The model under review builds one solid part; all positions refer to its coordinate system, in mm. Face numbers are marked on the shaded views. Coordinates: 2 decimals unless noted, no trailing zeros. Loops run counter-clockwise (first coordinate to the right, second up) from the corner with the lowest first, then second, coordinate; pieces in that order, holes last. Notation, with made-up numbers: (47, 83) - (65, 83) arc R13 cw to (65, 96) - close; hole circle Ø4 at (89.5, -3). An arc over 180 degrees is marked (long way). Answer in a Markdown table with one row per item. Add a question column.
(1) For P1, Ø5, axis at x = 28, z = 2.5, coming from the +Y side; P2, Ø4, axis at x = 67.5, y = 2.5, coming from the -Z side; P3, Ø2.5, axis at x = 20.5, y = 3, coming from the -Z side, all flat-tipped, find the tip position at first contact; note any pin that passes through.
(2) We need section B-B on x = 18. Write out the cut boundary in (y, z), plus the area to 3 significant figures.
(3) We need section A-A on z = -55. Write out the cut boundary in (x, y), plus the area to 3 significant figures.
(4) For line 1 along X through (y, z) = (0.75, -34); line 2 along X through (y, z) = (7, 6.5); line 3 along Y through (x, z) = (31.5, -3.5), list the stretches that pass through material, from the lowest coordinate up.
(5) Mouldability with a two-part tool opening along X and no side actions: class the marked faces 1 and 2 as +X half, -X half, draft (parallel to the pull), parting line (faces both ways), or undercut.
from build123d import *

# Parameters (mm, degrees)
EXTRUDE_4_DEPTH     = 5.6
EXTRUDE_4_2_DEPTH   = 5.6
SKETCH_9_W          = 2.6
SKETCH_9_H          = 12.4
SKETCH_9_H_2        = 50
EXTRUDE_6_DEPTH     = 2.6
DS18B20_W           = 5
DS18B20_H           = 42.5
DS18B20_H_2         = 10.1
CUT_EXTRUDE_1_DEPTH = 5
SKETCH_7_W          = 1.5
SKETCH_7_H          = 75
EXTRUDE_8_DEPTH     = 2.2
FILLET_1_RADIUS     = 4.7
FILLET_1_LENGTH     = 3
FILLET_2_R          = 7.3
FILLET_3_RADIUS     = 4.7
FILLET_3_LENGTH     = 3
FILLET_4_R          = 7.3
FILLET_5_RADIUS     = 4.7
FILLET_5_LENGTH     = 3
FILLET_6_R          = 7.3
FILLET_7_R          = 7.3
FILLET_8_RADIUS     = 4.7
FILLET_8_LENGTH     = 3
FILLET_9_RADIUS     = 4.7
FILLET_9_LENGTH     = 3
FILLET_10_R         = 7.3


with BuildPart() as part:
    # Sketch 2111 → Extrude 4 (new body)
    with BuildSketch(Plane(origin=(0, 0, 0), x_dir=(1, 0, 0), z_dir=(0, 1, 0))):
        Polygon((14.6, 50), (14.6, 0), (24, 0), (24, 50), (24, 52.6), (38.6, 52.6), (38.6, 50), (38.6, 0), (48, 0), (48, 50), (48, 52.6), (62.6, 52.6), (62.6, 50), (62.6, 0), (62.6, -12.4), (74.6, -12.4), (74.6, 62.6), (-12, 62.6), (-12, -12.4), (0, -12.4), (0, 0), (0, 50), (0, 52.6), (14.6, 52.6), align=None)
    extrude(amount=EXTRUDE_4_DEPTH)



with BuildPart() as body_2:
    # Sketch 2111 → Extrude 4 2 (new body)
    with BuildSketch(Plane(origin=(0, 0, 0), x_dir=(1, 0, 0), z_dir=(0, 1, 0))):
        Polygon((12, -2.6), (12, 0), (12, 50), (2.6, 50), (2.6, 0), (2.6, -12.4), (60, -12.4), (60, 0), (60, 50), (50.6, 50), (50.6, 0), (50.6, -2.6), (36, -2.6), (36, 0), (36, 50), (26.6, 50), (26.6, 0), (26.6, -2.6), align=None)
    extrude(amount=EXTRUDE_4_2_DEPTH)


with BuildPart() as part_1:
    add(part.part)

    add(body_2.part)  # Extrude 6 merges body 2
    # Sketch 9 → Extrude 6 (add)
    with BuildSketch(Plane(origin=(0, 0, 0), x_dir=(1, 0, 0), z_dir=(0, 1, 0))):
        with Locations((1.3, -6.2)):
            Rectangle(SKETCH_9_W, SKETCH_9_H)
        with Locations((1.3, 25)):
            Rectangle(SKETCH_9_W, SKETCH_9_H_2)
        Polygon((14.6, 0), (12, 0), (12, -2.6), (26.6, -2.6), (26.6, 0), (24, 0), align=None)
        with Locations((13.3, 25)):
            Rectangle(SKETCH_9_W, SKETCH_9_H_2)
        with Locations((25.3, 25)):
            Rectangle(SKETCH_9_W, SKETCH_9_H_2)
        Polygon((2.6, 50), (12, 50), (14.6, 50), (14.6, 52.6), (0, 52.6), (0, 50), align=None)
        Polygon((24, 52.6), (24, 50), (26.6, 50), (36, 50), (38.6, 50), (38.6, 52.6), align=None)
        with Locations((37.3, 25)):
            Rectangle(SKETCH_9_W, SKETCH_9_H_2)
        Polygon((38.6, 0), (36, 0), (36, -2.6), (50.6, -2.6), (50.6, 0), (48, 0), align=None)
        with Locations((49.3, 25)):
            Rectangle(SKETCH_9_W, SKETCH_9_H_2)
        Polygon((50.6, 50), (60, 50), (62.6, 50), (62.6, 52.6), (48, 52.6), (48, 50), align=None)
        with Locations((61.3, 25)):
            Rectangle(SKETCH_9_W, SKETCH_9_H_2)
        with Locations((61.3, -6.2)):
            Rectangle(SKETCH_9_W, SKETCH_9_H)
    extrude(amount=EXTRUDE_6_DEPTH)

    # DS18B20 → Cut-Extrude 1 (cut)
    with BuildSketch(Plane(origin=(0, 5.6, 0), x_dir=(1, 0, 0), z_dir=(0, 1, 0))):
        Polygon((-8.5, 62.6), (-8.5, 17.457748372), (-3.5, 19.012014035), (-3.5, 62.6), align=None)
        Polygon((-3.5, 19.012014035), (-8.5, 17.457748372), (-8.5, 10), (-3.5, 10), align=None)
        with Locations((19.3, 41.35)):
            Rectangle(DS18B20_W, DS18B20_H)
        with Locations((19.3, 15.05)):
            Rectangle(DS18B20_W, DS18B20_H_2)
        with Locations((43.3, 41.35)):
            Rectangle(DS18B20_W, DS18B20_H)
        with Locations((43.3, 15.05)):
            Rectangle(DS18B20_W, DS18B20_H_2)
        with Locations((68.6, 41.35)):
            Rectangle(DS18B20_W, DS18B20_H)
        with Locations((68.6, 15.05)):
            Rectangle(DS18B20_W, DS18B20_H_2)
    extrude(amount=-CUT_EXTRUDE_1_DEPTH, mode=Mode.SUBTRACT)

    # Sketch 7 → Extrude 8 (add)
    with BuildSketch(Plane(origin=(0, 5.6, 0), x_dir=(1, 0, 0), z_dir=(0, 1, 0))):
        with Locations((-11.25, 25.1)):
            Rectangle(SKETCH_7_W, SKETCH_7_H)
        with Locations((73.85, 25.1)):
            Rectangle(SKETCH_7_W, SKETCH_7_H)
    extrude(amount=EXTRUDE_8_DEPTH)

    # Fillet 1: full round fillet: the end face becomes a half cylinder, R = half its width
    fillet_1_face = Plane((55.3, 4.1, -50), x_dir=(0, -1, 0), z_dir=(0, 0, -1))  # on the end face: x along it, z out of the body
    fillet_1_slab = fillet_1_face.offset(-FILLET_1_RADIUS / 2) * Box(FILLET_1_LENGTH, 2 * FILLET_1_RADIUS, FILLET_1_RADIUS, mode=Mode.PRIVATE)  # the body's end, R deep
    fillet_1_round = Plane((55.3, 4.1, -45.3), x_dir=(0, 0, -1), z_dir=(0, -1, 0)) * Cylinder(FILLET_1_RADIUS, FILLET_1_LENGTH, mode=Mode.PRIVATE)  # its axis R under the face
    add(fillet_1_slab - fillet_1_round, mode=Mode.SUBTRACT)

    # Fillet 2
    fillet_2_edges = [part_1.edges().sort_by_distance(p)[0] for p in [
        (62.6, 4.1, -52.6),
        (48, 4.1, -52.6),
    ]]
    fillet(fillet_2_edges, radius=FILLET_2_R - 0.0001)  # a hair under: the kernel refuses the full size

    # Fillet 3: full round fillet: the end face becomes a half cylinder, R = half its width
    fillet_3_face = Plane((43.3, 4.1, 0), x_dir=(0, 1, 0), z_dir=(0, 0, 1))  # on the end face: x along it, z out of the body
    fillet_3_slab = fillet_3_face.offset(-FILLET_3_RADIUS / 2) * Box(FILLET_3_LENGTH, 2 * FILLET_3_RADIUS, FILLET_3_RADIUS, mode=Mode.PRIVATE)  # the body's end, R deep
    fillet_3_round = Plane((43.3, 4.1, -4.7), x_dir=(0, 0, 1), z_dir=(0, 1, 0)) * Cylinder(FILLET_3_RADIUS, FILLET_3_LENGTH, mode=Mode.PRIVATE)  # its axis R under the face
    add(fillet_3_slab - fillet_3_round, mode=Mode.SUBTRACT)

    # Fillet 4
    fillet_4_edges = [part_1.edges().sort_by_distance(p)[0] for p in [
        (50.6, 4.1, 2.6),
        (36, 4.1, 2.6),
    ]]
    fillet(fillet_4_edges, radius=FILLET_4_R - 0.0001)  # a hair under: the kernel refuses the full size

    # Fillet 5: full round fillet: the end face becomes a half cylinder, R = half its width
    fillet_5_face = Plane((31.3, 4.1, -50), x_dir=(0, -1, 0), z_dir=(0, 0, -1))  # on the end face: x along it, z out of the body
    fillet_5_slab = fillet_5_face.offset(-FILLET_5_RADIUS / 2) * Box(FILLET_5_LENGTH, 2 * FILLET_5_RADIUS, FILLET_5_RADIUS, mode=Mode.PRIVATE)  # the body's end, R deep
    fillet_5_round = Plane((31.3, 4.1, -45.3), x_dir=(0, 0, -1), z_dir=(0, -1, 0)) * Cylinder(FILLET_5_RADIUS, FILLET_5_LENGTH, mode=Mode.PRIVATE)  # its axis R under the face
    add(fillet_5_slab - fillet_5_round, mode=Mode.SUBTRACT)

    # Fillet 6
    fillet_6_edges = [part_1.edges().sort_by_distance(p)[0] for p in [
        (38.6, 4.1, -52.6),
        (24, 4.1, -52.6),
    ]]
    fillet(fillet_6_edges, radius=FILLET_6_R - 0.0001)  # a hair under: the kernel refuses the full size

    # Fillet 7
    fillet_7_edges = [part_1.edges().sort_by_distance(p)[0] for p in [
        (26.6, 4.1, 2.6),
        (12, 4.1, 2.6),
    ]]
    fillet(fillet_7_edges, radius=FILLET_7_R - 0.0001)  # a hair under: the kernel refuses the full size

    # Fillet 8: full round fillet: the end face becomes a half cylinder, R = half its width
    fillet_8_face = Plane((19.3, 4.1, 0), x_dir=(0, 1, 0), z_dir=(0, 0, 1))  # on the end face: x along it, z out of the body
    fillet_8_slab = fillet_8_face.offset(-FILLET_8_RADIUS / 2) * Box(FILLET_8_LENGTH, 2 * FILLET_8_RADIUS, FILLET_8_RADIUS, mode=Mode.PRIVATE)  # the body's end, R deep
    fillet_8_round = Plane((19.3, 4.1, -4.7), x_dir=(0, 0, 1), z_dir=(0, 1, 0)) * Cylinder(FILLET_8_RADIUS, FILLET_8_LENGTH, mode=Mode.PRIVATE)  # its axis R under the face
    add(fillet_8_slab - fillet_8_round, mode=Mode.SUBTRACT)

    # Fillet 9: full round fillet: the end face becomes a half cylinder, R = half its width
    fillet_9_face = Plane((7.3, 4.1, -50), x_dir=(0, 1, 0), z_dir=(0, 0, -1))  # on the end face: x along it, z out of the body
    fillet_9_slab = fillet_9_face.offset(-FILLET_9_RADIUS / 2) * Box(FILLET_9_LENGTH, 2 * FILLET_9_RADIUS, FILLET_9_RADIUS, mode=Mode.PRIVATE)  # the body's end, R deep
    fillet_9_round = Plane((7.3, 4.1, -45.3), x_dir=(0, 0, -1), z_dir=(0, 1, 0)) * Cylinder(FILLET_9_RADIUS, FILLET_9_LENGTH, mode=Mode.PRIVATE)  # its axis R under the face
    add(fillet_9_slab - fillet_9_round, mode=Mode.SUBTRACT)

    # Fillet 10
    fillet_10_edges = [part_1.edges().sort_by_distance(p)[0] for p in [
        (14.6, 4.1, -52.6),
        (0, 4.1, -52.6),
    ]]
    fillet(fillet_10_edges, radius=FILLET_10_R - 0.0001)  # a hair under: the kernel refuses the full size


solid = part_1.part
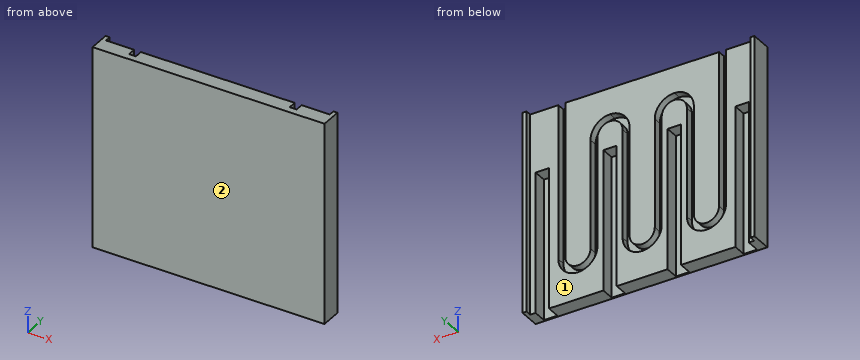
Outcome:
| question | item | result |
|---|---|---|
| 1 | P1 | y = 5.6 |
| 1 | P2 | z = -62.6 |
| 1 | P3 | z = -10 |
| 2 | outline | (0, -62.6) - (0.6, -62.6) - (0.6, -10) - (5.6, -10) - (5.6, -0.18) - (2.6, -0.18) - (2.6, 2.48) - (5.6, 2.48) - (5.6, 12.4) - (0, 12.4) - close |
| 2 | area | 149 mm² |
| 3 | outline | (-12, 0) - (74.6, 0) - (74.6, 7.8) - (73.1, 7.8) - (73.1, 5.6) - (71.1, 5.6) - (71.1, 0.6) - (66.1, 0.6) - (66.1, 5.6) - (45.8, 5.6) - (45.8, 0.6) - (40.8, 0.6) - (40.8, 5.6) - (21.8, 5.6) - (21.8, 0.6) - (16.8, 0.6) - (16.8, 5.6) - (-3.5, 5.6) - (-3.5, 0.6) - (-8.5, 0.6) - (-8.5, 5.6) - (-10.5, 5.6) - (-10.5, 7.8) - (-12, 7.8) - close |
| 3 | area | 392 mm² |
| 4 | line 1 | -12 to -8.5, -3.5 to 16.8, 21.8 to 40.8, 45.8 to 66.1, 71.1 to 74.6 |
| 4 | line 2 | -12 to -10.5, 73.1 to 74.6 |
| 4 | line 3 | 0 to 5.6 |
| 5 | face 1 | undercut |
| 5 | face 2 | draft |
